Source: three-view drawing plus pictorial views. Frame: mm from the lowest corner of the part. A direction names the side the tool comes from. Give positions to 0.01 mm unless a question says otherwise; leave off trailing zeros. Loops run counter-clockwise (first coordinate to the right, second up) from the corner with the lowest first, then second, coordinate; pieces in that order, holes last.
1. Section A-A, the plane x = 24.25. Output: boundary loops of the cut face in (y, z), then the cut area to 3 significant figures.
2. First-contact query: P1, Ø8, axis at x = 38.5, y = 14, coming from the -Z side; P2, Ø1.5, axis at x = 40.5, z = 10, coming from the -Y side; P3, Ø4, axis at y = 39, z = 17, coming from the -X side; P4, Ø10, axis at x = 7, z = 13, coming from the +Y side. Flat tips, straight axial feed; report the tip coordinate or a pass-through.
3. Access query for the marked faces 1 and 2. Directions: +Z, -Z, +X, -X, +Y, -Y. A direction counts if a zero-diameter tool reaches every point of the face in a straight line with its end or side. Return the directions, or none.
4. Material intervals for line 1 along Z through (x, y) = (46, 29.5); line 2 along Y through (x, z) = (43.5, 23); line 3 along Y through (x, z) = (21, 3.75), sorted ascending.
5. Section C-C, the plane z = 27.5. Output: boundary loops of the cut face in (x, y).
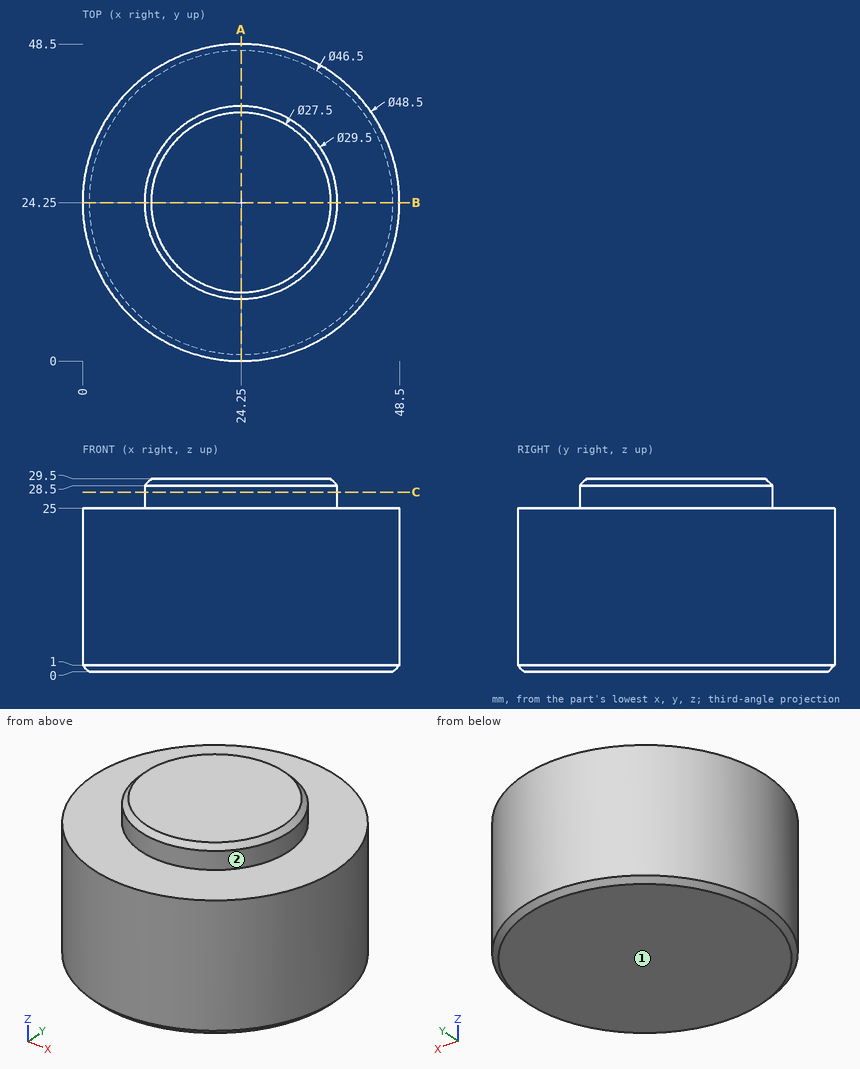
Answers below:
1. outline: (0, 1) - (1, 0) - (47.5, 0) - (48.5, 1) - (48.5, 25) - (39, 25) - (39, 28.5) - (38, 29.5) - (10.5, 29.5) - (9.5, 28.5) - (9.5, 25) - (0, 25) - close
1. area: 1,340 mm2
2. P1: stops at z = 0
2. P2: stops at y = 5.6
2. P3: stops at x = 3.62
2. P4: stops at y = 45.18
3. face 1: -Z, +X, -X, +Y, -Y
3. face 2: +Z
4. line 1: z = 0 to 25
4. line 2: y = 9.5 to 39
4. line 3: y = 0.22 to 48.28
5. outline: circle Ø29.5 at (24.25, 24.25)
